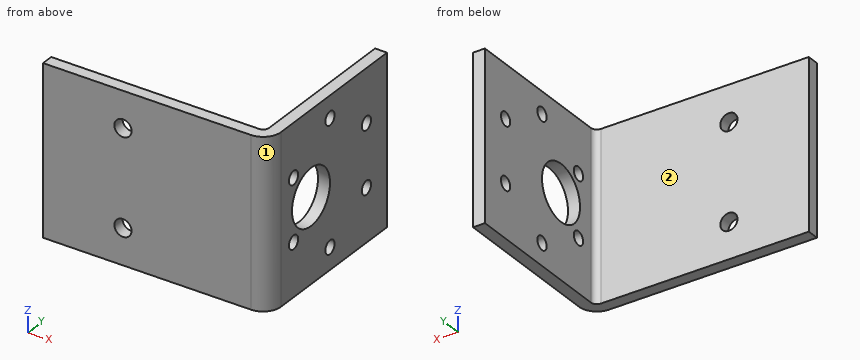
from build123d import *

# Parameters (mm, degrees)
SM_BRACKET_DEPTH     = 42
SK_MOTORHOLES_R      = 1.7
SK_MOTORHOLES_R_2    = 7
CUT_MOTORHOLES_DEPTH = 3
SK_RAILHOLES_R       = 2.15
CUT_RAILHOLES_DEPTH  = 30


# Sheet-metal steps are written as plain solids
with BuildPart() as part:
    # SK_Bracket → SM_Bracket (new body)
    with BuildSketch(Plane.XY.offset(-21)):
        with BuildLine():
            Line((0, 21), (0, -18))
            ThreePointArc((0, -18), (-0.439339828, -19.060660172), (-1.5, -19.5))
            Line((-1.5, -19.5), (-53.5, -19.5))
            Line((-53.5, -19.5), (-53.5, -22.5))
            Line((-53.5, -22.5), (-1.5, -22.5))
            ThreePointArc((-1.5, -22.5), (1.681980515, -21.181980515), (3, -18))
            Line((3, -18), (3, 21))
            Line((3, 21), (0, 21))
        make_face()
    extrude(amount=SM_BRACKET_DEPTH)

    # SK_MotorHoles → CUT_MotorHoles (cut)
    with BuildSketch(Plane(origin=(0, 0, 0), x_dir=(0, 0, -1), z_dir=(1, 0, 0))):
        with Locations((-15.5, 0)):
            Circle(SK_MOTORHOLES_R)
        with Locations((-7.75, 13.423393759)):
            Circle(SK_MOTORHOLES_R)
        with Locations((7.75, 13.423393759)):
            Circle(SK_MOTORHOLES_R)
        with Locations((15.5, 0)):
            Circle(SK_MOTORHOLES_R)
        with Locations((7.75, -13.423393759)):
            Circle(SK_MOTORHOLES_R)
        with Locations((-7.75, -13.423393759)):
            Circle(SK_MOTORHOLES_R)
        with Locations((0, -7)):
            Circle(SK_MOTORHOLES_R_2)
    extrude(amount=CUT_MOTORHOLES_DEPTH, mode=Mode.SUBTRACT)

    # SK_RailHoles → CUT_RailHoles (cut)
    with BuildSketch(Plane(origin=(0, 0, 0), x_dir=(1, 0, 0), z_dir=(0, 1, 0))):
        with Locations(Location((-33.5, -12, 0), (0, 0, 270))):
            Circle(SK_RAILHOLES_R)
        with Locations(Location((-33.5, 12, 0), (0, 0, 270))):
            Circle(SK_RAILHOLES_R)
    extrude(amount=-CUT_RAILHOLES_DEPTH, mode=Mode.SUBTRACT)


solid = part.part
Design review of the part built by this model. Coordinates are the model's own, in mm. Face numbers are marked on the shaded views. A direction names the side the tool comes from. Give positions to 0.01 mm unless a question says otherwise; leave off trailing zeros. Loops run counter-clockwise (first coordinate to the right, second up) from the corner with the lowest first, then second, coordinate; pieces in that order, holes last. Notation, with made-up numbers: M -21.75,-33 L 12.25,-33 A21 cw 12.25,4 Z; hole C 7,12 d4. An arc over 180 degrees is marked long. Answer as a JSON object with one key per item and string values.
Item 1: Machinability: for the marked faces 1 and 2, which of the approach directions +Z, -Z, +X, -X, +Y, -Y give a long, thin tool a straight path to every point of the face, cutting with its end or side? Answer none if there is none.
Output values:
{"face 1": "+Z, -Z, +X, -Y", "face 2": "+Z, -Z, -X, +Y"}
Item 2: For P1, Ø8, axis at x = -9, z = -3.5, coming from the +Y side; P2, Ø3, axis at y = -13.42, z = 7.75, coming from the +X side; P3, Ø10, axis at y = 0.5, z = -3.5, coming from the -X side, all flat-tipped, find the tip position at first contact; note any pin that passes through.
Output values:
{"P1": "stops at y = -19.5", "P2": "passes through", "P3": "stops at x = 0"}
Item 3: We need section A-A (z = 0). State the section outline as (x, y) points, and give its area (3 significant figures).
Output values:
{"outline": "M -53.5,-22.5 L -1.5,-22.5 A4.5 ccw 3,-18 L 3,-14 L 0,-14 L 0,-18 A1.5 cw -1.5,-19.5 L -53.5,-19.5 Z; M 0,0 L 3,0 L 3,21 L 0,21 Z", "area": "245 mm2"}
Item 4: We need section C-C (y = 1). State the section outline as (x, z) points.
Output values:
{"outline": "M 0,-21 L 3,-21 L 3,-16.87 L 0,-16.87 Z; M 0,-14.13 L 3,-14.13 L 3,14.13 L 0,14.13 Z; M 0,16.87 L 3,16.87 L 3,21 L 0,21 Z"}
Item 5: We need section B-B (z = -7.75). State the section outline as (x, y) points, and give its area (3 significant figures).
Output values:
{"outline": "M -53.5,-22.5 L -1.5,-22.5 A4.5 ccw 3,-18 L 3,-15.12 L 0,-15.12 L 0,-18 A1.5 cw -1.5,-19.5 L -53.5,-19.5 Z; M 0,-11.72 L 3,-11.72 L 3,11.72 L 0,11.72 Z; M 0,15.12 L 3,15.12 L 3,21 L 0,21 Z", "area": "267 mm2"}
Item 6: We need section D-D (y = -9). State the section outline as (x, z) points.
Output values:
{"outline": "M 0,-21 L 3,-21 L 3,-6.71 L 0,-6.71 Z; M 0,6.71 L 3,6.71 L 3,21 L 0,21 Z"}
Item 7: Wall thickness on line 1 along Y through (x, z) = (1.3, 7.75); line 2 along Y through (x, z) = (-1.5, -12); line 3 along X through (y, z) = (15, 16.5): over which ranges is each line inside the solid? List them lowest first.
Output values:
{"line 1": "y = -21.52 to -15.12, -11.72 to 11.72, 15.12 to 21", "line 2": "y = -22.5 to -19.5", "line 3": "x = 0 to 3"}
